Check sheet for the modelled part. Datum: model origin and axes. Units: mm. Face numbers are marked on the shaded views. A direction names the side the tool comes from. Give positions to 0.01 mm unless a question says otherwise; leave off trailing zeros. Loops run counter-clockwise (first coordinate to the right, second up) from the corner with the lowest first, then second, coordinate; pieces in that order, holes last. Notation, with made-up numbers: (42, 65.25) -> (57, 65.25) arc R21 ccw to (57, 73.25) -> close; hole circle Ø6 at (28.5, 19.25). An arc over 180 degrees is marked (long way). Answer as CSV lines item,"result". Start each with the question number.
(1) Section check B-B on z = -24. Enter the section's corners in (x, y), plus the area to 3 significant figures.
(2) Material ranges on line 1 (Y direction, x = 7.75, z = -24); line 2 (Y direction, x = 10, z = -22.5); line 3 (Z direction, x = -2.75, y = 2.25), recorded low to high. Write a range as from..to.
(3) Section check C-C on y = 5.75. Enter the section's corners in (x, z), plus the area to 3 significant figures.
(4) Section check D-D on y = 0. Enter the section's corners in (x, z).
(5) Access from +Z, -Z, +X, -X, +Y, -Y to the whole of each face (thin tool, end or side, straight path). Record for the marked faces 1 and 2.
(6) Gauge pin test, flat ends, axial feed: pin 1 Ø2 at (y, z) = (3.5, 6.5) entering from +X; pin 2 Ø2 at (x, z) = (-7.5, -21.5) entering from -Y; pin 3 Ø2 at (y, z) = (0, 3) entering from +X; pin 4 Ø12 at (y, z) = (-8.5, -14) entering from -X. Record the tip position at first contact, or that the pin passes through.
(7) Section check A-A on x = 0. Enter the section's corners in (y, z).
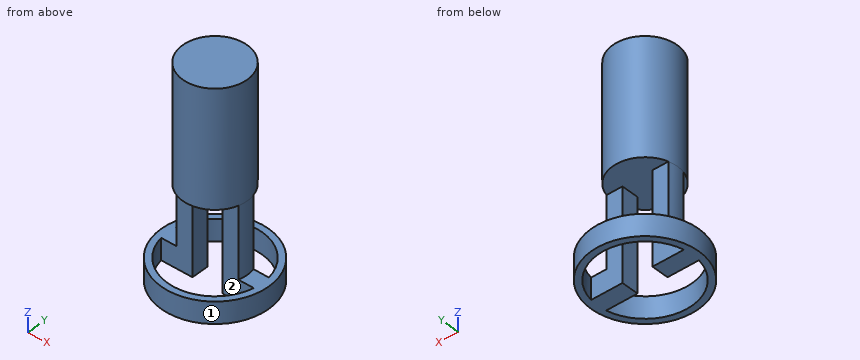
from build123d import *

# Parameters (mm, degrees)
SKETCH_R     = 7.5
PAD_DEPTH    = 9
SKETCH001_R  = 7.5
PAD001_DEPTH = 2
SKETCH002_R  = 7.5
PAD002_DEPTH = 9
SKETCH003_R  = 7.5
PAD003_DEPTH = 1.5
SKETCH004_R  = 7.5
PAD004_DEPTH = 5.5
PAD005_DEPTH = 21.5
SKETCH006_R  = 12.5
PAD006_DEPTH = 5


with BuildPart() as part:
    # Sketch → Pad (new body)
    with BuildSketch(Plane.XY):
        Circle(SKETCH_R)
    extrude(amount=PAD_DEPTH)

    # Sketch001 (on Face3 of Pad) → Pad001 (join)
    with BuildSketch(Plane.XY.offset(9)):
        Circle(SKETCH001_R)
    extrude(amount=PAD001_DEPTH)

    # Sketch002 (on Face4 of Pad001) → Pad002 (join)
    with BuildSketch(Plane.XY.offset(11)):
        Circle(SKETCH002_R)
    extrude(amount=PAD002_DEPTH)

    # Sketch003 (on Face5 of Pad002) → Pad003 (join)
    with BuildSketch(Plane.XY.offset(20)):
        Circle(SKETCH003_R)
    extrude(amount=PAD003_DEPTH)

    # Sketch004 (on Face2 of Pad003) → Pad004 (join)
    with BuildSketch(Plane(origin=(0, 0, 0), x_dir=(1, 0, 0), z_dir=(0, 0, -1))):
        Circle(SKETCH004_R)
    extrude(amount=PAD004_DEPTH)

    # Sketch005 (on Face4 of Pad004) → Pad005 (join)
    with BuildSketch(Plane(origin=(0, 0, -5.5), x_dir=(1, 0, 0), z_dir=(0, 0, -1))):
        with BuildLine():
            Line((3.5, 2), (3.5, -2))
            Line((3.5, -2), (7.228416, -2))
            ThreePointArc((7.228416, -2), (7.5, 0), (7.228416, 2))
            Line((3.5, 2), (7.228416, 2))
        make_face()
        with BuildLine():
            Line((-3.5, 2), (-3.5, -2))
            Line((-3.5, -2), (-7.228416, -2))
            ThreePointArc((-7.228416, 2), (-7.5, 0), (-7.228416, -2))
            Line((-3.5, 2), (-7.228416, 2))
        make_face()
    extrude(amount=PAD005_DEPTH)

    # Sketch006 (on Face15 of Pad005) → Pad006 (join)
    with BuildSketch(Plane(origin=(0, 0, -27), x_dir=(1, 0, 0), z_dir=(0, 0, -1))):
        Circle(SKETCH006_R)
        with BuildLine():
            ThreePointArc((10.816654, 2), (0, 11), (-10.816654, 2))
            Line((-3.5, 2), (-10.816654, 2))
            Line((-3.5, -2), (-3.5, 2))
            Line((-10.816654, -2), (-3.5, -2))
            ThreePointArc((-10.816654, -2), (0, -11), (10.816654, -2))
            Line((10.816654, -2), (3.5, -2))
            Line((3.5, -2), (3.5, 2))
            Line((3.5, 2), (10.816654, 2))
        make_face(mode=Mode.SUBTRACT)
    extrude(amount=-PAD006_DEPTH)


solid = part.part
Working result:
1,outline,"circle Ø25 at (0, 0); hole (-10.82, -2) arc R11 ccw to (10.82, -2) -> (3.5, -2) -> (3.5, 2) -> (10.82, 2) arc R11 ccw to (-10.82, 2) -> (-3.5, 2) -> (-3.5, -2) -> close"
1,area,"170 mm^2"
2,line 1,"y = -9.81..-7.81, -2..2, 7.81..9.81"
2,line 2,"y = -7.5..-4.58, -2..2, 4.58..7.5"
2,line 3,"z = -5.5..21.5"
3,outline,"(-11.1, -27) -> (-9.38, -27) -> (-9.38, -22) -> (-11.1, -22) -> close; (-4.82, -5.5) -> (4.82, -5.5) -> (4.82, 21.5) -> (-4.82, 21.5) -> close; (9.38, -27) -> (11.1, -27) -> (11.1, -22) -> (9.38, -22) -> close"
3,area,"277 mm^2"
4,outline,"(-12.5, -27) -> (-3.5, -27) -> (-3.5, -5.5) -> (3.5, -5.5) -> (3.5, -27) -> (12.5, -27) -> (12.5, -22) -> (7.5, -22) -> (7.5, 21.5) -> (-7.5, 21.5) -> (-7.5, -22) -> (-12.5, -22) -> close"
5,face 1,"+Z, -Z"
5,face 2,"-Z"
6,pin 1,"stops at x = 7.07"
6,pin 2,"stops at y = -10.59"
6,pin 3,"stops at x = 7.5"
6,pin 4,"passes through"
7,outline,"(-12.5, -27) -> (-11, -27) -> (-11, -22) -> (-12.5, -22) -> close; (-7.5, -5.5) -> (7.5, -5.5) -> (7.5, 21.5) -> (-7.5, 21.5) -> close; (11, -27) -> (12.5, -27) -> (12.5, -22) -> (11, -22) -> close"
